Design review of the part built by this model. Coordinates are the model's own, in mm. Face numbers are marked on the shaded views. A direction names the side the tool comes from. Coordinates: 2 decimals unless noted, no trailing zeros. Loops run counter-clockwise (first coordinate to the right, second up) from the corner with the lowest first, then second, coordinate; pieces in that order, holes last. Notation, with made-up numbers: (-23.75, 44.25) -> (-0.75, 44.25) arc R14 cw to (-0.75, 65.25) -> close; hole circle Ø3 at (-20.5, 84.25). An arc over 180 degrees is marked (long way). Answer as a JSON object with one key per item and string values.
```python
from build123d import *

# Parameters (mm, degrees)
SKETCH_1_W          = 60
SKETCH_1_H          = 24
EXTRUDE_1_DEPTH     = 22
SKETCH_3_W          = 24
SKETCH_3_H          = 20
CUT_EXTRUDE_2_DEPTH = 18
SKETCH_5_W          = 13
SKETCH_5_H          = 16
CUT_EXTRUDE_4_DEPTH = 4
SKETCH_6_W          = 24
SKETCH_6_H          = 20
CUT_EXTRUDE_5_DEPTH = 5


with BuildPart() as part:
    # ｽｹｯﾁ1 → ﾎﾞｽ - 押し出し1 (new body)
    with BuildSketch(Plane.XY):
        Rectangle(SKETCH_1_W, SKETCH_1_H)
    extrude(amount=EXTRUDE_1_DEPTH)

    # ｽｹｯﾁ3 → ｶｯﾄ - 押し出し2 (cut)
    with BuildSketch(Plane.XY.offset(22)):
        with Locations((-15, 0)):
            Rectangle(SKETCH_3_W, SKETCH_3_H)
    cut_extrude_2 = extrude(amount=-CUT_EXTRUDE_2_DEPTH, mode=Mode.SUBTRACT)

    # ｽｹｯﾁ5 → ｶｯﾄ - 押し出し4 (cut)
    with BuildSketch(Plane.XY.offset(4)):
        with Locations((-15, 4)):
            Rectangle(SKETCH_5_W, SKETCH_5_H)
    cut_extrude_4 = extrude(amount=-CUT_EXTRUDE_4_DEPTH, mode=Mode.SUBTRACT)

    # ｽｹｯﾁ6 → ｶｯﾄ - 押し出し5 (cut)
    with BuildSketch(Plane(origin=(0, 12, 0), x_dir=(1, 0, 0), z_dir=(0, 1, 0))):
        with Locations((-15, -12)):
            Rectangle(SKETCH_6_W, SKETCH_6_H)
    cut_extrude_5 = extrude(amount=-CUT_EXTRUDE_5_DEPTH, mode=Mode.SUBTRACT)

    # ﾐﾗｰ1: ｶｯﾄ - 押し出し2, ｶｯﾄ - 押し出し4, ｶｯﾄ - 押し出し5 across plane
    add(cut_extrude_2.mirror(Plane(origin=(0, 0, 0), x_dir=(0, 0, 1), z_dir=(1, 0, 0))), mode=Mode.SUBTRACT)
    add(cut_extrude_4.mirror(Plane(origin=(0, 0, 0), x_dir=(0, 0, 1), z_dir=(1, 0, 0))), mode=Mode.SUBTRACT)
    add(cut_extrude_5.mirror(Plane(origin=(0, 0, 0), x_dir=(0, 0, 1), z_dir=(1, 0, 0))), mode=Mode.SUBTRACT)


solid = part.part
```
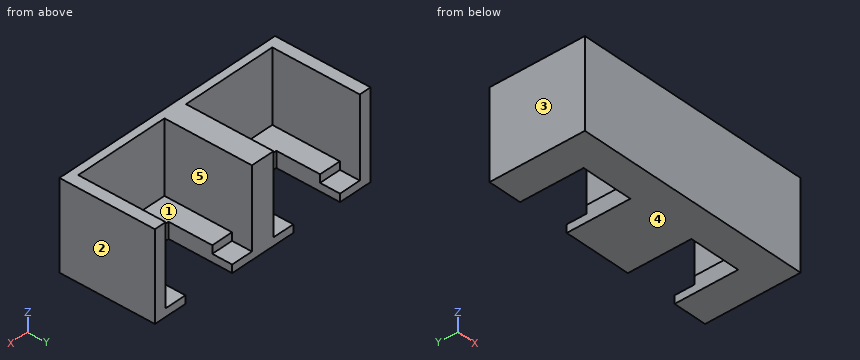
1) Add section A-A, the plane y = 4.75. Give the boundary of the cut face in (x, z).
Completed:
{"outline": "(-30, 0) -> (-21.5, 0) -> (-21.5, 4) -> (-27, 4) -> (-27, 22) -> (-30, 22) -> close; (-8.5, 0) -> (8.5, 0) -> (8.5, 4) -> (3, 4) -> (3, 22) -> (-3, 22) -> (-3, 4) -> (-8.5, 4) -> close; (21.5, 0) -> (30, 0) -> (30, 22) -> (27, 22) -> (27, 4) -> (21.5, 4) -> close"}
2) Clearance check with flat-ended pins moving along their axes: pin 1 Ø1.5 at (x, y) = (23.5, 10.5) entering from +Z; pin 2 Ø3 at (x, z) = (-14, 2) entering from +Y; pin 3 Ø5.5 at (x, y) = (-23.5, 9.5) entering from +Z. State where each tip first meets the part, or that it passes through.
Completed:
{"pin 1": "z = 2", "pin 2": "y = -4", "pin 3": "z = 4"}
3) Wall thickness on probe 1 along X at (y, z) = (1, 10.25); probe 2 along Y at (x, z) = (-17, 16.75); probe 3 along Z at (x, y) = (13.5, -8): over which ranges is each line inside the solid? List them lowest first.
Completed:
{"probe 1": "-30 to -27, -3 to 3, 27 to 30", "probe 2": "-12 to -10", "probe 3": "0 to 4"}
4) The part is to be moulded in two halves that separate along X. For the marked faces 3, 4 and 5, say which applies: pulls with the +X half, pulls with the -X half, needs draft (parallel to the pull), parting line crosses it, or undercut.
Completed:
{"face 3": "pulls with the -X half", "face 4": "needs draft", "face 5": "undercut"}
5) Add section C-C, the plane x = 23.5. Give the boundary of the cut face in (y, z).
Completed:
{"outline": "(-12, 0) -> (12, 0) -> (12, 2) -> (7, 2) -> (7, 4) -> (-10, 4) -> (-10, 22) -> (-12, 22) -> close"}
6) For the marked faces 1 and 2, list the 3-axis set-ups (+Z, -Z, +X, -X, +Y, -Y) from which the entire face can be reached by the end or side of a thin tool; tool diameter is ignored.
Completed:
{"face 1": "+Z, +Y", "face 2": "+Z, -Z, +X, +Y, -Y"}
7) Add section B-B, the plane z = 10.25. Give the boundary of the cut face in (x, y).
Completed:
{"outline": "(-30, -12) -> (30, -12) -> (30, 12) -> (27, 12) -> (27, -10) -> (3, -10) -> (3, 12) -> (-3, 12) -> (-3, -10) -> (-27, -10) -> (-27, 12) -> (-30, 12) -> close"}
8) Add section D-D, the plane y = 8. Give the boundary of the cut face in (x, z).
Completed:
{"outline": "(-30, 0) -> (-21.5, 0) -> (-21.5, 2) -> (-27, 2) -> (-27, 22) -> (-30, 22) -> close; (-8.5, 0) -> (8.5, 0) -> (8.5, 2) -> (3, 2) -> (3, 22) -> (-3, 22) -> (-3, 2) -> (-8.5, 2) -> close; (21.5, 0) -> (30, 0) -> (30, 22) -> (27, 22) -> (27, 2) -> (21.5, 2) -> close"}
